Could you check a few things on this model? Use its own coordinates, in mm. A direction names the side the tool comes from. Coordinates: 2 decimals unless noted, no trailing zeros. Loops run counter-clockwise (first coordinate to the right, second up) from the corner with the lowest first, then second, coordinate; pieces in that order, holes last. Notation, with made-up numbers: (66, 42) - (81, 42) arc R22 cw to (81, 67) - close; hole circle Ø11 at (73, 50). An arc over 180 degrees is marked (long way). Use CSV: the item, a comma, the result in double quotes.
from build123d import *

# Parameters (mm, degrees)
SKETCH_1_W               = 50
SKETCH_1_H               = 55
EXTRUDE_1_DEPTH          = 2
SKETCH_2_R               = 1.5
CUT_EXTRUDE_1_DEPTH      = 3
CUT_EXTRUDE_2_DEPTH      = 10
CUT_EXTRUDE_3_DEPTH      = 20.5
CUT_EXTRUDE_3_DEPTH_BACK = 36.5
SKETCH_5_R               = 1.75
CUT_EXTRUDE_4_DEPTH      = 10
CUT_EXTRUDE_5_DEPTH      = 10
SKETCH_7_R               = 2.5
CUT_EXTRUDE_6_DEPTH      = 10
FILLET_1_R               = 2


with BuildPart() as part:
    # 草图1 → 凸台-拉伸1 (new body)
    with BuildSketch(Plane(origin=(0, 0, 0), x_dir=(1, 0, 0), z_dir=(0, 1, 0))):
        Rectangle(SKETCH_1_W, SKETCH_1_H)
    extrude(amount=EXTRUDE_1_DEPTH)

    # 草图2 → 切除-拉伸1 (cut, through all)
    with BuildSketch(Plane(origin=(0, 2, 0), x_dir=(1, 0, 0), z_dir=(0, 1, 0))):
        with Locations((-18, 8)):
            Circle(SKETCH_2_R)
        with Locations((-18, -8)):
            Circle(SKETCH_2_R)
        with Locations((12, -8)):
            Circle(SKETCH_2_R)
        with Locations((12, 8)):
            Circle(SKETCH_2_R)
    extrude(amount=-CUT_EXTRUDE_1_DEPTH, mode=Mode.SUBTRACT)

    # 草图3 → 切除-拉伸2 (cut)
    with BuildSketch(Plane.XZ):
        with BuildLine():
            Line((-18, 9.5), (-15, 9.5))
            ThreePointArc((-15, 9.5), (-13.5, 8), (-15, 6.5))
            Line((-15, 6.5), (-18, 6.5))
            Line((-18, 6.5), (-18, 9.5))
        make_face()
    cut_extrude_2 = extrude(amount=-CUT_EXTRUDE_2_DEPTH, mode=Mode.SUBTRACT)

    # 草图4 → 切除-拉伸3 (cut, two sides)
    with BuildSketch(Plane.XY.offset(8)) as cut_extrude_3_sk:
        Polygon((-18, 0), (-15, 0.315312706), (-15, 0), align=None)
    extrude(amount=CUT_EXTRUDE_3_DEPTH, mode=Mode.SUBTRACT)
    extrude(cut_extrude_3_sk.sketch, amount=-CUT_EXTRUDE_3_DEPTH_BACK, mode=Mode.SUBTRACT)

    # 镜向1: 切除-拉伸2 across plane
    add(cut_extrude_2.mirror(Plane.XY), mode=Mode.SUBTRACT)

    # 草图5 → 切除-拉伸4 (cut)
    with BuildSketch(Plane(origin=(0, 2, 0), x_dir=(1, 0, 0), z_dir=(0, 1, 0))):
        with Locations((20, 21)):
            Circle(SKETCH_5_R)
        with Locations((20, -21)):
            Circle(SKETCH_5_R)
    extrude(amount=-CUT_EXTRUDE_4_DEPTH, mode=Mode.SUBTRACT)

    # 草图6 → 切除-拉伸5 (cut)
    with BuildSketch(Plane(origin=(0, 2, 0), x_dir=(1, 0, 0), z_dir=(0, 1, 0))):
        Polygon((-25, 17.5), (0, 17.5), (17.320508076, 27.5), (-25, 27.5), align=None)
        Polygon((17.320508076, -27.5), (-25, -27.5), (-25, -17.5), (0, -17.5), align=None)
    extrude(amount=-CUT_EXTRUDE_5_DEPTH, mode=Mode.SUBTRACT)

    # 草图7 → 切除-拉伸6 (cut)
    with BuildSketch(Plane.XZ):
        with Locations((-5.685574087, -11.419607443)):
            Circle(SKETCH_7_R)
        with Locations((-0.540616532, -2.844678186)):
            Circle(SKETCH_7_R)
        with Locations((-4.144957554, 12.343977362)):
            Circle(SKETCH_7_R)
        with Locations((1, 3.769048105)):
            Circle(SKETCH_7_R)
    extrude(amount=-CUT_EXTRUDE_6_DEPTH, mode=Mode.SUBTRACT)

    # 圆角1
    fillet_1_edges = [part.edges().sort_by_distance(p)[0] for p in [
        (17.320508076, 1, -27.5),
        (-25, 1, -17.5),
        (0, 1, -17.5),
        (0, 1, 17.5),
        (17.320508076, 1, 27.5),
        (-25, 1, 17.5),
        (25, 1, 27.5),
        (25, 1, -27.5),
    ]]
    fillet(fillet_1_edges, radius=FILLET_1_R)


solid = part.part
(1) Thinking about a two-plate mould opening in X: for faces 1 (the face through (-24.43, 0.99, 16.9)), 2 (the face through (24.4, 1.01, -26.93)), 3 (the face through (18.71, 1.01, 19.82)), which applies, +X half, -X half, draft (parallel to the pull), parting line (faces both ways), or undercut?
Computed:
face 1,"-X half"
face 2,"+X half"
face 3,"undercut"
(2) Suppose I cut it at D-D (x = -12). Write out the boundary of the cut face in (y, z).
Computed:
outline,"(0, -17.5) - (2, -17.5) - (2, 17.5) - (0, 17.5) - close"
(3) Suppose I cut it at C-C (z = 21). Write out the boundary of the cut face in (x, y).
Computed:
outline,"(6.06, 0) - (18.25, 0) - (18.25, 2) - (6.06, 2) - close; (21.75, 0) - (25, 0) - (25, 2) - (21.75, 2) - close"
(4) Please list where these lines run through material, in increasing order: line 1 (X direction, y = 1.25, z = -8); line 2 (Z direction, x = 20, y = 1.65); line 3 (Z direction, x = -17, y = 0.45).
Computed:
line 1,"x = -25 to -19.5, -13.5 to 10.5, 13.5 to 25"
line 2,"z = -27.5 to -22.75, -19.25 to 19.25, 22.75 to 27.5"
line 3,"z = -17.5 to -9.5, -6.5 to 6.5, 9.5 to 17.5"
(5) Which directions (+Z, -Z, +X, -X, +Y, -Y) give clear straight access to the entire face, cutting with the end or side of a thin tool? Please do faces 4 (the face through (-16.521, 0.155, 0.091)), 5 (the face through (-12, 1, 17.5)), 6 (the face through (-13.5, 1, -8)), 7 (the face through (-12, 1, -17.5)).
Computed:
face 4,"+Z, -Z, -Y"
face 5,"+Z, -X, +Y, -Y"
face 6,"+Y, -Y"
face 7,"-Z, -X, +Y, -Y"
(6) Suppose I cut it at A-A (x = 20). Write out the boundary of the cut face in (y, z), plus the area to 3 significant figures.
Computed:
outline,"(0, -27.5) - (2, -27.5) - (2, -22.75) - (0, -22.75) - close; (0, -19.25) - (2, -19.25) - (2, 19.25) - (0, 19.25) - close; (0, 22.75) - (2, 22.75) - (2, 27.5) - (0, 27.5) - close"
area,"96.0 mm²"
(7) Suppose I cut it at B-B (z = -8). Write out the boundary of the cut face in (x, y).
Computed:
outline,"(-25, 0) - (-19.5, 0) - (-19.5, 2) - (-25, 2) - close; (-13.5, 0) - (10.5, 0) - (10.5, 2) - (-13.5, 2) - close; (13.5, 0) - (25, 0) - (25, 2) - (13.5, 2) - close"
(8) Will these pins go through, and if not, where does the flat tip stop? pin 1 (2 mm diameter, centred on x = 14.5, z = 13.5, fed in from -Y); pin 2 (2.5 mm diameter, centred on x = 12, z = -8, fed in from -Y); pin 3 (1 mm diameter, centred on x = -16, y = 0.5, fed in from -Z).
Computed:
pin 1,"stops at y = 0"
pin 2,"passes through"
pin 3,"stops at z = -17.5"
